```python
from build123d import *

# Parameters (mm, degrees)
DODANIE_WYCI_GNI_CIE1_DEPTH = 10
SZKIC2_R                    = 1.5
DODANIE_WYCI_GNI_CIE2_DEPTH = 5
SFAZOWANIE2_SIZE            = 0.5
OTW_R_GWINTOWANY_M31_D      = 2.5
OTW_R_GWINTOWANY_M31_DEPTH  = 8
OTW_R_GWINTOWANY_M31_TIP    = 0.751075774
SFAZOWANIE3_SIZE            = 0.1
SZKIC29_R                   = 0.91230631
WYTNIJ_WYCI_GNI_CIE1_DEPTH  = 12.814539066


with BuildPart() as part:
    # Szkic1 → Dodanie-wyciągnięcie1 (new body)
    with BuildSketch(Plane.XY):
        Polygon((0, 2.886751346), (-2.5, 1.443375673), (-2.5, -1.443375673), (0, -2.886751346), (2.5, -1.443375673), (2.5, 1.443375673), align=None)
    extrude(amount=DODANIE_WYCI_GNI_CIE1_DEPTH)

    # Szkic2 → Dodanie-wyciągnięcie2 (add)
    with BuildSketch(Plane(origin=(0, 0, 0), x_dir=(-1, 0, 0), z_dir=(0, 0, -1))):
        with Locations(Location((0, 0, 0), (0, 0, 180))):
            Circle(SZKIC2_R)
    extrude(amount=DODANIE_WYCI_GNI_CIE2_DEPTH)

    # Sfazowanie2
    sfazowanie2_edges = [part.edges().sort_by_distance(p)[0] for p in [
        (-1.5, 0, -5),
    ]]
    chamfer(sfazowanie2_edges, length=SFAZOWANIE2_SIZE)

    # Otwór gwintowany M31
    with Locations(Plane.XY.offset(10)):
        with Locations((0, 0)):
            Hole(OTW_R_GWINTOWANY_M31_D / 2, depth=OTW_R_GWINTOWANY_M31_DEPTH)
            with Locations((0, 0, -(OTW_R_GWINTOWANY_M31_DEPTH + OTW_R_GWINTOWANY_M31_TIP / 2))):  # 118° drill point
                Cone(0, OTW_R_GWINTOWANY_M31_D / 2, OTW_R_GWINTOWANY_M31_TIP, mode=Mode.SUBTRACT)

    # Sfazowanie3
    sfazowanie3_edges = [part.edges().sort_by_distance(p)[0] for p in [
        (-2.5, 0, 10),
        (-1.25, -2.165063509, 10),
        (1.25, -2.165063509, 10),
        (2.5, 0, 10),
        (1.25, 2.165063509, 10),
        (2.5, 0, 0),
        (1.25, -2.165063509, 0),
        (-1.25, -2.165063509, 0),
        (-1.25, 2.165063509, 10),
        (-2.5, 0, 0),
        (-1.25, 2.165063509, 0),
        (1.25, 2.165063509, 0),
    ]]
    chamfer(sfazowanie3_edges, length=SFAZOWANIE3_SIZE)

    # Szkic29 → Wytnij-wyciągnięcie1 (cut, through all)
    with BuildSketch(Plane(origin=(1.25, 2.165063509, 0), x_dir=(0.8660254037844415, -0.49999999999999517, 0), z_dir=(0.4999999999999951, 0.8660254037844414, 0))):
        with Locations(Location((0, -5.034184195, 0), (0, 0, 180))):
            Circle(SZKIC29_R)
    extrude(amount=-WYTNIJ_WYCI_GNI_CIE1_DEPTH, mode=Mode.SUBTRACT)


solid = part.part
```
Check sheet for the modelled part. Datum: model origin and axes. Units: mm. A direction names the side the tool comes from. Give positions to 0.01 mm unless a question says otherwise; leave off trailing zeros. Write each loop counter-clockwise with the first axis right and the second up, starting at its lowest first coordinate (ties: lowest second). Pieces come first, ordered by that corner, then holes. Notation, with made-up numbers: (52.5, -10) - (86.5, -10) arc R31 cw to (86.5, 20) - close; hole circle Ø4 at (20.5, 28). An arc over 180 degrees is marked (long way). Answer as a JSON object with one key per item and string values. Group by question number.
1) Depth check by flat-ended pin: P1, Ø1.5, axis at x = 0.5, z = 6, coming from the -Y side. Enter the tip coordinate at first touch or a pass-through.
2) Access from +Z, -Z, +X, -X, +Y, -Y to the whole of each face (thin tool, end or side, straight path). Record for faces 1 (the face through (-2, 0, 0)), 2 (the face through (-1.65, -1.18, 4.68)).
3) Sectioned sample at A-A (z = -3.5). Record the cut outline in (x, y).
4) Release check for a two-part mould opening along Y. For faces 3 (the face through (-1.233, 2.175, 4.931)), 4 (the face through (-1.267, -2.155, 3.843)), 5 (the face through (1.25, 0.05, 5.94)), 6 (the face through (-1, -1, 10)) record: pulls with the +Y half, pulls with the -Y half, needs draft (parallel to the pull), parting line crosses it, or undercut.
5) Thickness scan on probe 1 along X at (y, z) = (0, 5); probe 2 along X at (y, z) = (-1.5, 0.75); probe 3 along Y at (x, z) = (0.35, 9). Record the ranges inside material, lowest first. Write a range as from..to.
Geometry results:
{
 "1": {"P1": "stops at y = -2.89"},
 "2": {"face 1": "-Z", "face 2": "none"},
 "3": {"outline": "circle Ø3 at (0, 0)"},
 "4": {"face 3": "pulls with the +Y half", "face 4": "pulls with the -Y half", "face 5": "undercut", "face 6": "needs draft"},
 "5": {"probe 1": "x = -2.5..-1.25, 1.25..2.5", "probe 2": "x = -2.4..2.4", "probe 3": "y = -2.68..-1.2, 1.2..2.68"}
}
